Autodesk Inventor part; units mm, degrees
ref_plane "YZ Plane" through (0, 0, 0) normal (1, 0, 0) x (0, 1, 0)
ref_plane "XZ Plane" through (0, 0, 0) normal (0, 1, 0) x (-1, 0, 0)
ref_plane "XY Plane" through (0, 0, 0) normal (0, 0, 1) x (1, 0, 0)
sketch "Sketch1" plane through (0, 0, 0) normal (1, 0, 0) x (0, 1, 0)
  line L0 (0, 0) -> (0, 56)
  line L1 (-11.5, 56) -> (-11.5, 2.5)
  line L2 (-11.5, 2.5) -> (-13, 2.5)
  line L3 (-13, 2.5) -> (-13, 0)
  line L4 (-13, 0) -> (-20, 0)
  line L5 (-20, 0) -> (-20, 3)
  line L6 (-20, 3) -> (-13.5, 4.7417)
  line L7 (-13.5, 4.7417) -> (-13.5, 44.7417)
  line L8 (-13.5, 44.7417) -> (-13, 44.7417)
  line L9 (-13, 44.7417) -> (-13, 56)
  line L10 (-13, 56) -> (-11.5, 56)
  dimension "d0" = 56
  dimension "d1" = 27
  dimension "d2" = 26
  dimension "d3" = 2.5
  dimension "d4" = 23
  dimension "d5" = 15
  dimension "d6" = 3
  dimension "d7" = 40
  dimension "d8" = 26
  dimension "d10" = 40
revolve "Revolution1" add sketch "Sketch1" angle 360 about axis through (0, 0, 0) along (0, 0, 1)
fillet "Fillet1" radius 1 2 edges at (0, 20, 3) (0, 13.5, 4.7417)
sketch "Sketch2" plane through (0, 0, 0) normal (1, 0, 0) x (0, 1, 0)
  circle A0 centre (0, 80) radius 28.5
  line L0 (20, 0) -> (-20, 0)
  point P0 (0, 0)
  dimension "d13" = 57
  dimension "d14" = 80
extrude "Extrusion1" cut sketch "Sketch2" along normal through all both and the other way through all
chamfer "Chamfer1" distance 0.2 angle 45 4 edges at (0, 20, 0) (0, 13, 0) (0, 11.5, 2.5) (0, 13, 2.5)
properties part number "pld_vessel_kf_nipple" material "Stainless Steel"
Model file for the job. Use its own axes, mm. A direction names the side the tool comes from. Round coordinates to 2 decimals unless told otherwise and drop trailing zeros. Write each loop counter-clockwise with the first axis right and the second up, starting at its lowest first coordinate (ties: lowest second). Pieces come first, ordered by that corner, then holes. Notation, with made-up numbers: M 74,52 L 81,52 A30 cw 81,81 Z; hole C 67.25,-30 d6. An arc over 180 degrees is marked long. Put each result on its own line as item: value.
Item 1: Cut at A-A (z = 41). List the corners of the cut face in (x, y).
Responses:
outline: C 0,0 d27; hole C 0,0 d23
Item 2: Probe L1, parallel to X at y = 0, z = 39; L2, parallel to X at y = 0, z = 1.1. List the from-to ranges inside material, lowest first. Write a range as from..to.
Responses:
L1: -13.5..-11.5, 11.5..13.5
L2: -20..-13, 13..20
Item 3: Cut at B-B (z = 46.5). List the corners of the cut face in (x, y), and give its area (3 significant figures).
Responses:
outline: C 0,0 d26; hole C 0,0 d23
area: 115 mm²
Item 4: Flat gauge pins, fed straight in: P1, Ø8, axis at x = -5, z = 33.5, coming from the +Y side; P2, Ø1, axis at x = 10, z = 39.5, coming from the -Y side; P3, Ø10, axis at x = 2.5, z = 42.5, coming from the -Y side. Where does each tip first touch, or does it go through?
Responses:
P1: y = 13.46
P2: y = -9.59
P3: y = -13.5
Item 5: Tool access for faces 1 (the flat face through (-3.7, -11.3, 2.5)), 2 (the cylindrical face through (8.79, 9.58, 48.66)), 3 (the cylindrical face through (6.007, -19.076, 1.231)): list every direction of +Z, -Z, +X, -X, +Y, -Y with a clear straight run to the whole face (end or side of a thin tool).
Responses:
face 1: -Z
face 2: +Z
face 3: +Z, -Z
